Verification items for this drawing (mm, ordinates from the low corner). Coordinates: 2 decimals unless noted, no trailing zeros. Write each loop counter-clockwise with the first axis right and the second up, starting at its lowest first coordinate (ties: lowest second). Pieces come first, ordered by that corner, then holes. Notation, with made-up numbers: (38, -18) -> (44, -18) arc R11 cw to (44, -9) -> close; hole circle Ø9 at (40, 10.5). An arc over 180 degrees is marked (long way). One line per question, with ' | ' between items.
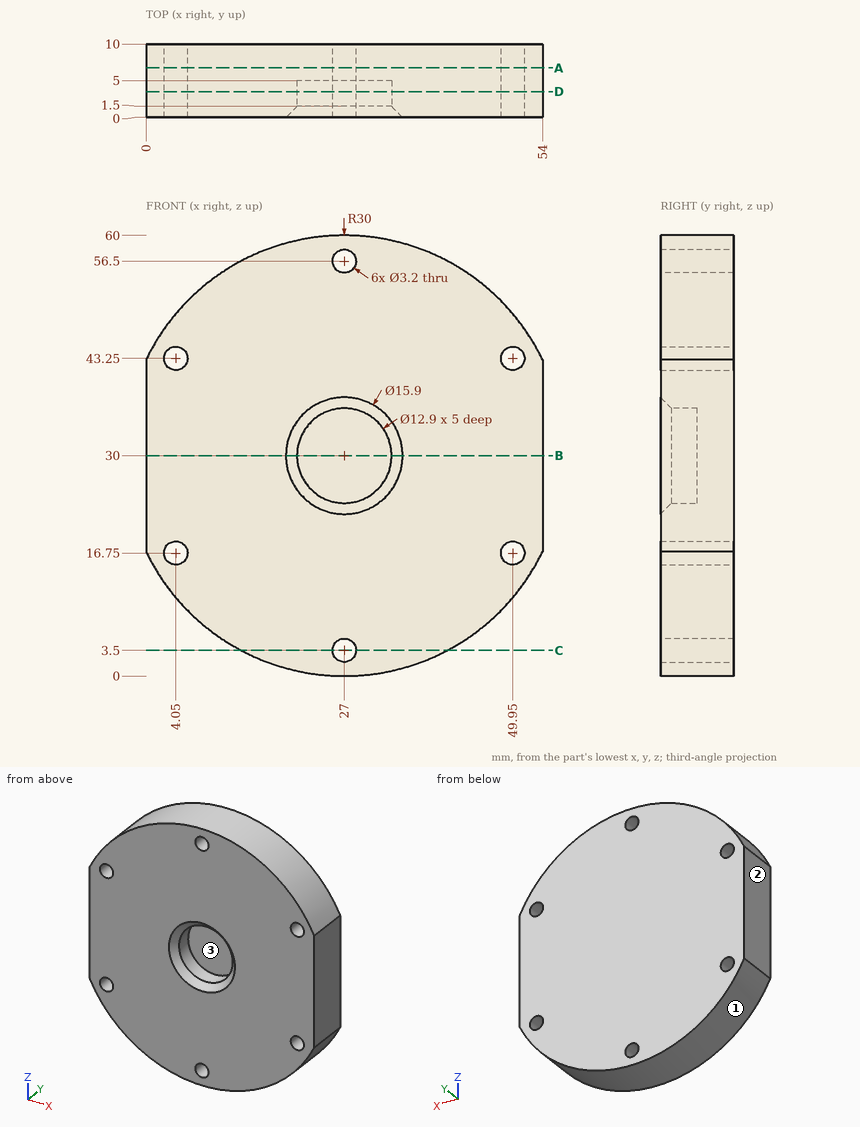
(1) Cross-section at D-D (y = 3.5). Record the cut outline in (x, z), plus the area to 3 significant figures.
Answers below:
outline: (0, 16.92) arc R30 ccw to (54, 16.92) -> (54, 43.08) arc R30 ccw to (0, 43.08) -> close; hole circle Ø3.2 at (4.05, 16.75); hole circle Ø3.2 at (4.05, 43.25); hole circle Ø12.9 at (27, 30); hole circle Ø3.2 at (27, 3.5); hole circle Ø3.2 at (27, 56.5); hole circle Ø3.2 at (49.95, 16.75); hole circle Ø3.2 at (49.95, 43.25) | area: 2,540 mm²
(2) Cross-section at A-A (y = 6.75). Record the cut outline in (x, z), plus the area to 3 significant figures.
Answers below:
outline: (0, 16.92) arc R30 ccw to (54, 16.92) -> (54, 43.08) arc R30 ccw to (0, 43.08) -> close; hole circle Ø3.2 at (4.05, 16.75); hole circle Ø3.2 at (4.05, 43.25); hole circle Ø3.2 at (27, 3.5); hole circle Ø3.2 at (27, 56.5); hole circle Ø3.2 at (49.95, 16.75); hole circle Ø3.2 at (49.95, 43.25) | area: 2,670 mm²
(3) Depth check by flat-ended pin: P1, Ø2, axis at y = 8.5, z = 36, coming from the -X side; P2, Ø3, axis at x = 8, y = 2, coming from the +Z side; P3, Ø5, axis at x = 27, y = 7.5, coming from the +Z side. Enter the tip coordinate at first touch or a pass-through.
Answers below:
P1: stops at x = 0 | P2: stops at z = 54.37 | P3: stops at z = 60
(4) Draft check along Z on the marked faces 1, 2 and 3. Enter one of: pulls with the +Z half, pulls with the -Z half, needs draft (parallel to the pull), parting line crosses it, or undercut.
Answers below:
face 1: pulls with the -Z half | face 2: needs draft | face 3: undercut
(5) Cross-section at C-C (z = 3.5). Record the cut outline in (x, y).
Answers below:
outline: (12.94, 0) -> (25.4, 0) -> (25.4, 10) -> (12.94, 10) -> close; (28.6, 0) -> (41.06, 0) -> (41.06, 10) -> (28.6, 10) -> close
(6) Material ranges on line 1 (X direction, y = 2.3, z = 30); line 2 (Z direction, x = 48.5, y = 2.75) (1 decimal); line 3 (X direction, y = 0.75, z = 31), recorded low to high.
Answers below:
line 1: x = 0 to 20.55, 33.45 to 54 | line 2: z = 9.1 to 16.1, 17.4 to 42.6, 43.9 to 50.9 | line 3: x = 0 to 19.87, 34.13 to 54
(7) Cross-section at B-B (z = 30). Record the cut outline in (x, y).
Answers below:
outline: (0, 0) -> (19.05, 0) -> (20.55, 1.5) -> (20.55, 5) -> (33.45, 5) -> (33.45, 1.5) -> (34.95, 0) -> (54, 0) -> (54, 10) -> (0, 10) -> close
